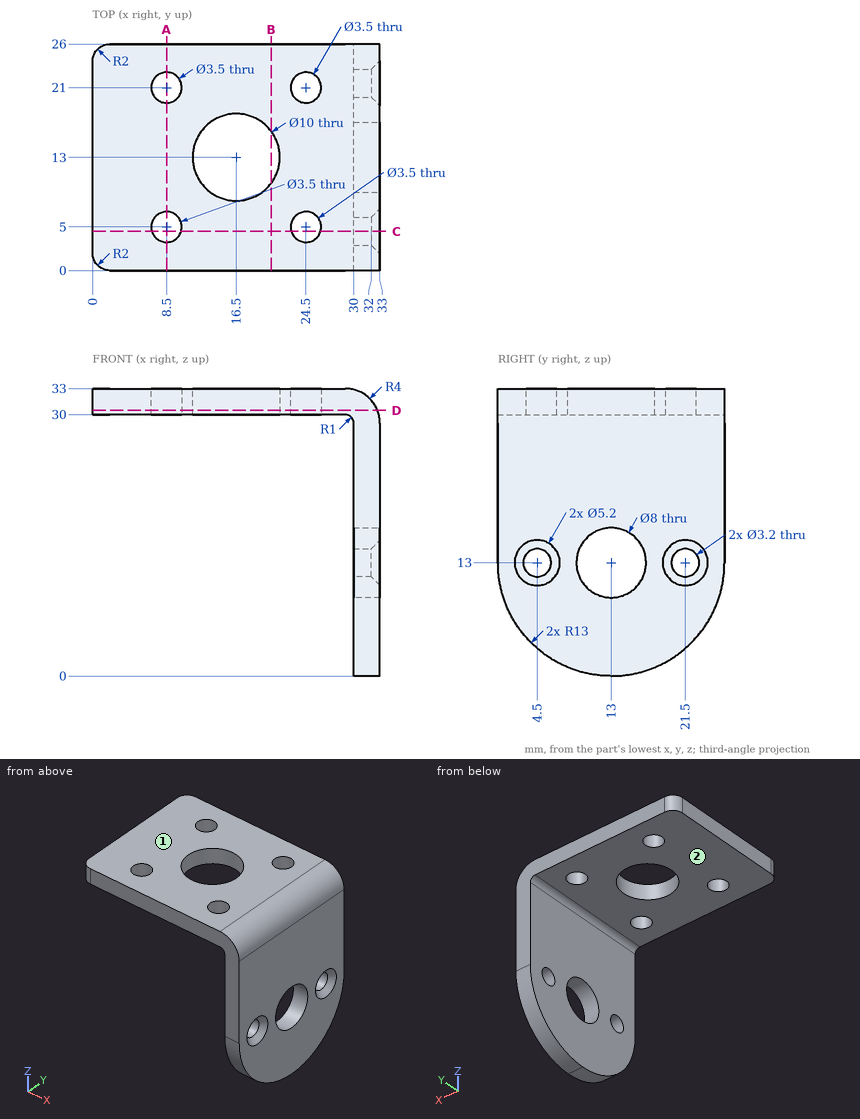
Could you check a few things on this drawing? It's one solid part, dimensions in mm from its lowest x, y, z. A direction names the side the tool comes from. Coordinates: 2 decimals unless noted, no trailing zeros. Order: outer loops, then holes, each group sorted by start corner. A loop starts at its lowest first (then second) coordinate and runs counter-clockwise, first axis right, second up. Notation, with made-up numbers: (22, 71.25) - (61, 71.25) arc R32 cw to (61, 97.25) - close; hole circle Ø5 at (-12.75, 51.25). An arc over 180 degrees is marked (long way). One line per question, with ' | ' between items.
(1) Suppose I cut it at A-A on x = 8.5. List the corners of the cut face in (y, z) for me, and give its area (3 significant figures).
Report:
outline: (0, 30) - (3.25, 30) - (3.25, 33) - (0, 33) - close; (6.75, 30) - (19.25, 30) - (19.25, 33) - (6.75, 33) - close; (22.75, 30) - (26, 30) - (26, 33) - (22.75, 33) - close | area: 57.0 mm2
(2) Will these pins go through, and if not, where does the flat tip stop? pin 1 (4 mm diameter, centred on x = 24.5, y = 5, fed in from -Z); pin 2 (4 mm diameter, centred on y = 22.5, z = 7.5, fed in from -X); pin 3 (4 mm diameter, centred on y = 4.5, z = 13, fed in from +X).
Report:
pin 1: stops at z = 30 | pin 2: stops at x = 30 | pin 3: stops at x = 32.4
(3) If I drill on L1, parallel to Y at x = 30.7, z = 13; L2, parallel to X at y = 3.25, z = 7.5, over which ranges is the centre line in solid material (lowest first)?
Report:
L1: y = 0 to 2.9, 6.1 to 9, 17 to 19.9, 23.1 to 26 | L2: x = 30 to 33
(4) For the marked faces 1 and 2, which set-ups out of +Z, -Z, +X, -X, +Y, -Y let a thin tool reach every point of the face, with its end or its side?
Report:
face 1: +Z, +X, -X, +Y, -Y | face 2: -Z, -X, +Y, -Y
(5) Suppose I cut it at C-C on y = 4.5. List the corners of the cut face in (x, z) for me.
Report:
outline: (0, 30) - (6.82, 30) - (6.82, 33) - (0, 33) - close; (10.18, 30) - (22.82, 30) - (22.82, 33) - (10.18, 33) - close; (26.18, 30) - (29, 30) arc R1 cw to (30, 29) - (30, 14.6) - (32, 14.6) - (33, 15.6) - (33, 29) arc R4 ccw to (29, 33) - (26.18, 33) - close; (30, 3.16) - (33, 3.16) - (33, 10.4) - (32, 11.4) - (30, 11.4) - close
(6) Suppose I cut it at D-D on z = 30.5. List the corners of the cut face in (x, y) for me, and give its area (3 significant figures).
Report:
outline: (0, 2) arc R2 ccw to (2, 0) - (32.71, 0) - (32.71, 26) - (2, 26) arc R2 ccw to (0, 24) - close; hole circle Ø3.5 at (8.5, 5); hole circle Ø3.5 at (8.5, 21); hole circle Ø10 at (16.5, 13); hole circle Ø3.5 at (24.5, 5); hole circle Ø3.5 at (24.5, 21) | area: 732 mm2
(7) Suppose I cut it at B-B on x = 20.5. List the corners of the cut face in (y, z) for me.
Report:
outline: (0, 30) - (10, 30) - (10, 33) - (0, 33) - close; (16, 30) - (26, 30) - (26, 33) - (16, 33) - close
